from build123d import *

# Parameters (mm, degrees)
SCHIZZO1_W                   = 66
SCHIZZO1_H                   = 85
ESTRUSIONE_ESTRUSIONE1_DEPTH = 20
RACCORDO1_R                  = 5
RACCORDO2_R                  = 5
RACCORDO3_R                  = 5
SVUOTA2_T                    = -1.5
SCHIZZO3_R                   = 0.5
ESTRUSIONE_ESTRUSIONE2_DEPTH = 15
SCHIZZO6_R                   = 0.5
ESTRUSIONE_ESTRUSIONE3_DEPTH = 15
SCHIZZO13_W                  = 25
SCHIZZO13_H                  = 10
TAGLIO_ESTRUSIONE2_DEPTH     = 2
SCHIZZO19_W                  = 46
SCHIZZO19_H                  = 10
TAGLIO_ESTRUSIONE5_DEPTH     = 2
ESTRUSIONE_ESTRUSIONE4_DEPTH = 3
SCHIZZO18_W                  = 48.51759383
SCHIZZO18_H                  = 2
TAGLIO_ESTRUSIONE6_DEPTH     = 80
SCHIZZO22_W                  = 25
SCHIZZO22_H                  = 10
TAGLIO_ESTRUSIONE7_DEPTH     = 2


with BuildPart() as part:
    # Schizzo1 → Estrusione-Estrusione1 (new body)
    with BuildSketch(Plane(origin=(0, 0, 0), x_dir=(1, 0, 0), z_dir=(0, 1, 0))):
        with Locations((33, 42.5)):
            Rectangle(SCHIZZO1_W, SCHIZZO1_H)
    extrude(amount=ESTRUSIONE_ESTRUSIONE1_DEPTH)

    # Raccordo1
    raccordo1_edges = [part.edges().sort_by_distance(p)[0] for p in [
        (66, 10, 0),
        (0, 10, 0),
    ]]
    fillet(raccordo1_edges, radius=RACCORDO1_R)

    # Raccordo2
    raccordo2_edges = [part.edges().sort_by_distance(p)[0] for p in [
        (66, 10, -85),
    ]]
    fillet(raccordo2_edges, radius=RACCORDO2_R)

    # Raccordo3
    raccordo3_edges = [part.edges().sort_by_distance(p)[0] for p in [
        (0, 10, -85),
    ]]
    fillet(raccordo3_edges, radius=RACCORDO3_R)

    # Svuota2
    svuota2_openings = [part.faces().sort_by_distance(p)[0] for p in [
        (33, 20, -42.5),
    ]]
    offset(amount=SVUOTA2_T, openings=svuota2_openings, kind=Kind.INTERSECTION)

    # Schizzo3 → Estrusione-Estrusione2 (add)
    with BuildSketch(Plane(origin=(0, 1.5, 0), x_dir=(1, 0, 0), z_dir=(0, 1, 0))):
        with Locations(Location((5.5, 77.89, 0), (0, 0, 90))):
            Circle(SCHIZZO3_R)
    extrude(amount=ESTRUSIONE_ESTRUSIONE2_DEPTH)

    # Schizzo6 → Estrusione-Estrusione3 (add)
    with BuildSketch(Plane(origin=(0, 1.5, 0), x_dir=(1, 0, 0), z_dir=(0, 1, 0))):
        with Locations(Location((58.664950896, 77.535960271, 0), (0, 0, 90))):
            Circle(SCHIZZO6_R)
        with Locations(Location((58.664950896, 5.132828607, 0), (0, 0, 90))):
            Circle(SCHIZZO6_R)
        with Locations(Location((5.345748971, 5.132828607, 0), (0, 0, 90))):
            Circle(SCHIZZO6_R)
    extrude(amount=ESTRUSIONE_ESTRUSIONE3_DEPTH)

    # Schizzo13 → Taglio-Estrusione2 (cut)
    with BuildSketch(Plane(origin=(0, 0, -85), x_dir=(-1, 0, 0), z_dir=(0, 0, -1))):
        with Locations((-42.5, 9)):
            Rectangle(SCHIZZO13_W, SCHIZZO13_H)
    extrude(amount=-TAGLIO_ESTRUSIONE2_DEPTH, mode=Mode.SUBTRACT)

    # Schizzo19 → Taglio-Estrusione5 (cut)
    with BuildSketch(Plane.XY):
        with Locations((33, 9)):
            Rectangle(SCHIZZO19_W, SCHIZZO19_H)
    extrude(amount=-TAGLIO_ESTRUSIONE5_DEPTH, mode=Mode.SUBTRACT)

    # Schizzo21 → Estrusione-Estrusione4 (add)
    with BuildSketch(Plane.XZ):
        with BuildLine():
            Line((5, 0), (61, 0))
            ThreePointArc((61, 0), (64.535533906, -1.464466094), (66, -5))
            Line((66, -5), (66, -80))
            ThreePointArc((66, -80), (64.535533906, -83.535533906), (61, -85))
            Line((61, -85), (5, -85))
            ThreePointArc((5, -85), (1.464466094, -83.535533906), (0, -80))
            Line((0, -80), (0, -5))
            ThreePointArc((0, -5), (1.464466094, -1.464466094), (5, 0))
        make_face()
    extrude(amount=ESTRUSIONE_ESTRUSIONE4_DEPTH)

    # Schizzo18 → Taglio-Estrusione6 (cut)
    with BuildSketch(Plane.ZY):
        with Locations((-42.307961204, -1.3)):
            Rectangle(SCHIZZO18_W, SCHIZZO18_H)
    extrude(amount=-TAGLIO_ESTRUSIONE6_DEPTH, mode=Mode.SUBTRACT)

    # Schizzo22 → Taglio-Estrusione7 (cut)
    with BuildSketch(Plane(origin=(66, 0, 0), x_dir=(0, 0, -1), z_dir=(1, 0, 0))):
        with Locations((42.5, 7.5)):
            Rectangle(SCHIZZO22_W, SCHIZZO22_H)
    extrude(amount=-TAGLIO_ESTRUSIONE7_DEPTH, mode=Mode.SUBTRACT)


solid = part.part
The listing builds one solid part. Answer for the finished solid, in the listing's coordinates (mm). A direction names the side the tool comes from. Give positions to 0.01 mm unless a question says otherwise; leave off trailing zeros. Write each loop counter-clockwise with the first axis right and the second up, starting at its lowest first coordinate (ties: lowest second). Pieces come first, ordered by that corner, then holes.
Item 1: Section C-C, the plane z = -51 is taken. Write down the section's boundary in (x, y), plus the area to 4 significant figures.
Item 2: Determine the mould class of faces 1 (the flat face through (66, 14, -42)), 2 (the flat face through (27, 9, -85)), 3 (the flat face through (1.5, 11, -42)), 4 (the flat face through (26, 11, -83.5)) for opening direction X: released by +X, released by -X, zero draft, split by the parting line, or undercut.
Item 3: Find the intervals of material crossed by line 1 along X through (y, z) = (8.25, -27); line 2 along Z through (x, y) = (27.5, 16.5); line 3 along Y through (x, z) = (19.5, -20), in increasing order.
Item 4: Flat-ended cylindrical pins translate along their axes: P1, Ø1.6, axis at x = 65, y = 9, coming from the -Z side; P2, Ø0.8, axis at y = 9, z = -84.5, coming from the +X side; P3, Ø0.8, axis at x = 5.5, z = -78, coming from the +Y side. Find the tip coordinate at first contact, or state that the pin passes through.
Item 5: Section B-B, the plane z = -22 is taken. Write down the section's boundary in (x, y).
Item 6: Section A-A, the plane x = 23 is taken. Write down the section's boundary in (y, z).
Item 7: Section D-D, the plane z = -72 is taken. Write down the section's boundary in (x, y), plus the area to 4 significant figures.
Item 8: Which of the six approach directions +Z, -Z, +X, -X, +Y, -Y give full straight-line access (tool end or side, diameter ignored) to faces 5 (the flat face through (33, -1, -18.049)), 6 (the flat face through (33, 1.5, -43)), 7 (the flat face through (32.6, 3.5, 0))?
Completed:
1. outline: (0, -3) - (66, -3) - (66, -2.3) - (0, -2.3) - close; (0, -0.3) - (66, -0.3) - (66, 2.5) - (64.5, 2.5) - (64.5, 1.5) - (1.5, 1.5) - (1.5, 20) - (0, 20) - close; (64.5, 12.5) - (66, 12.5) - (66, 20) - (64.5, 20) - close
1. area: 205.5 mm2
2. face 1: released by +X
2. face 2: zero draft
2. face 3: undercut
2. face 4: undercut
3. line 1: x = 0 to 1.5, 64.5 to 66
3. line 2: z = -85 to -83.5, -1.5 to 0
3. line 3: y = -3 to -2.3, -0.3 to 1.5
4. P1: stops at z = -83.84
4. P2: stops at x = 63.86
4. P3: stops at y = 16.5
5. outline: (0, -3) - (66, -3) - (66, -2.3) - (0, -2.3) - close; (0, -0.3) - (66, -0.3) - (66, 20) - (64.5, 20) - (64.5, 1.5) - (1.5, 1.5) - (1.5, 20) - (0, 20) - close
6. outline: (-3, -85) - (20, -85) - (20, -83.5) - (1.5, -83.5) - (1.5, -1.5) - (4, -1.5) - (4, 0) - (-3, 0) - close; (14, -1.5) - (20, -1.5) - (20, 0) - (14, 0) - close; hole (-2.3, -66.57) - (-0.3, -66.57) - (-0.3, -18.05) - (-2.3, -18.05) - close
7. outline: (0, -3) - (66, -3) - (66, 20) - (64.5, 20) - (64.5, 1.5) - (1.5, 1.5) - (1.5, 20) - (0, 20) - close
7. area: 352.5 mm2
8. face 5: +X, -X
8. face 6: +Y
8. face 7: +Z, +X, -X, +Y, -Y
